from build123d import *

# Parameters (mm, degrees)
F0_W     = 31.75
F0_H     = 31.75
F0_W_2   = 9.525
F0_H_2   = 50.8
F0_R     = 3.175
F0_R_2   = 6.35
F1_DEPTH = 12.7
F2_R     = 3.175
F3_W     = 9.525
F3_H     = 38.1
F4_DEPTH = 1.5875
F5_W     = 9.525
F5_H     = 12.7
F6_DEPTH = 1.5875
F7_W     = 9.525
F7_H     = 50.8
F8_DEPTH = 1.5875
F9_R     = 6.35


with BuildPart() as f1:
    # F0 (on Right) → F1 (new body)
    with BuildSketch(Plane.YZ):
        with BuildLine():
            Line((0, 41.275), (0, 0))
            Line((0, 0), (130.175, 0))
            Line((130.175, 0), (130.175, 50.8))
            Line((130.175, 50.8), (73.025, 50.8))
            Line((73.025, 50.8), (73.025, 44.45))
            ThreePointArc((73.025, 44.45), (76.2, 41.275), (73.025, 38.1))
            Line((73.025, 38.1), (63.5, 38.1))
            ThreePointArc((63.5, 38.1), (60.325, 41.275), (63.5, 44.45))
            Line((63.5, 44.45), (63.5, 50.8))
            Line((63.5, 50.8), (50.8, 50.8))
            Line((50.8, 50.8), (50.8, 25.4))
            ThreePointArc((50.8, 25.4), (44.45, 19.05), (38.1, 25.4))
            Line((38.1, 25.4), (38.1, 50.8))
            Line((38.1, 50.8), (26.7157145118, 50.8))
            Line((26.7157145118, 50.8), (0, 41.275))
        make_face()
        with Locations((104.775, 25.4)):
            Rectangle(F0_W, F0_H, mode=Mode.SUBTRACT)
        with Locations((134.9375, 25.4)):
            Rectangle(F0_W_2, F0_H_2)
        with BuildLine():
            Line((139.7, 50.8), (139.7, 0))
            Line((139.7, 0), (304.8, 0))
            Line((304.8, 0), (304.8, 19.05))
            Line((304.8, 19.05), (266.7, 19.05))
            Line((266.7, 19.05), (266.7, 40.9178125))
            Line((266.7, 40.9178125), (290.922752809, 52.7264044944))
            ThreePointArc((290.922752809, 52.7264044944), (299.6985955056, 78.197752809), (274.227247191, 86.9735955056))
            Line((274.227247191, 86.9735955056), (200.025, 50.8))
            Line((200.025, 50.8), (139.7, 50.8))
        make_face()
        with Locations((230.1875, 12.7)):
            Circle(F0_R, mode=Mode.SUBTRACT)
        with Locations((165.1, 25.4)):
            Rectangle(F0_W, F0_H, mode=Mode.SUBTRACT)
        with BuildLine():
            Line((190.5, 38.1), (200.025, 38.1))
            ThreePointArc((200.025, 38.1), (203.2, 34.925), (200.025, 31.75))
            Line((200.025, 31.75), (200.025, 19.05))
            ThreePointArc((200.025, 19.05), (203.2, 15.875), (200.025, 12.7))
            Line((200.025, 12.7), (190.5, 12.7))
            ThreePointArc((190.5, 12.7), (187.325, 15.875), (190.5, 19.05))
            Line((190.5, 19.05), (190.5, 31.75))
            ThreePointArc((190.5, 31.75), (187.325, 34.925), (190.5, 38.1))
        make_face(mode=Mode.SUBTRACT)
        with Locations((282.575, 69.85)):
            Circle(F0_R_2, mode=Mode.SUBTRACT)
    extrude(amount=F1_DEPTH)

    # F2
    f2_edges = [f1.edges().sort_by_distance(p)[0] for p in [
        (6.35, 200.025, 50.8),
        (6.35, 266.7, 40.917812),
        (6.35, 266.7, 19.05),
        (6.35, 304.8, 19.05),
        (6.35, 304.8, 0),
    ]]
    fillet(f2_edges, radius=F2_R)

    # F3 (on face) → F4 (cut)
    with BuildSketch(Plane.YZ.offset(12.7)):
        with Locations((68.2625, 19.05)):
            Rectangle(F3_W, F3_H)
    extrude(amount=-F4_DEPTH, mode=Mode.SUBTRACT)

    # F5 (on face) → F6 (cut)
    with BuildSketch(Plane.YZ.offset(12.7)):
        with Locations((195.2625, 6.35)):
            Rectangle(F5_W, F5_H)
        with BuildLine():
            ThreePointArc((199.2923076923, 50.8), (199.6611512097, 50.8214972713), (200.025, 50.8856979781))
            Line((200.025, 50.8856979781), (200.025, 52.109055835))
            Line((200.025, 52.109055835), (190.5, 52.109055835))
            Line((190.5, 52.109055835), (190.5, 50.8))
            Line((190.5, 50.8), (199.2923076923, 50.8))
        make_face()
        with BuildLine():
            Line((190.5, 38.1), (200.025, 38.1))
            Line((200.025, 38.1), (200.025, 50.8856979781))
            ThreePointArc((200.025, 50.8856979781), (199.6611512097, 50.8214972713), (199.2923076923, 50.8))
            Line((199.2923076923, 50.8), (190.5, 50.8))
            Line((190.5, 50.8), (190.5, 38.1))
        make_face()
    extrude(amount=-F6_DEPTH, mode=Mode.SUBTRACT)

    # F7 (on face) → F8 (cut)
    with BuildSketch(Plane.YZ.offset(12.7)):
        with Locations((134.9375, 25.4)):
            Rectangle(F7_W, F7_H)
    extrude(amount=-F8_DEPTH, mode=Mode.SUBTRACT)

    # F9
    f9_edges = [f1.edges().sort_by_distance(p)[0] for p in [
        (6.35, 88.9, 41.275),
        (6.35, 120.65, 41.275),
        (6.35, 180.975, 41.275),
        (6.35, 149.225, 41.275),
        (6.35, 149.225, 9.525),
        (6.35, 88.9, 9.525),
        (6.35, 180.975, 9.525),
        (6.35, 120.65, 9.525),
    ]]
    fillet(f9_edges, radius=F9_R)


solid = f1.part
Design review of the part built by this model. Coordinates are the model's own, in mm. A direction names the side the tool comes from. Coordinates: 2 decimals unless noted, no trailing zeros. Order: outer loops, then holes, each group sorted by start corner. A loop starts at its lowest first (then second) coordinate and runs counter-clockwise, first axis right, second up.
Item 1: Take a section at A-A, the plane y = 166.5. Write out the cut boundary in (x, z) (3 decimals).
Item 2: For line 1 (Z direction, x = 7.25, y = 175); line 2 (Z direction, x = 9, y = 62.5); line 3 (Y direction, x = 5.25, z = 72), list the stretches that pass through material, from the lowest coordinate up.
Item 3: For pin 1 Ø4 at (x, z) = (9, 63.5) entering from +Y; pin 2 Ø0.5 at (x, z) = (12, 28) entering from +Y; pin 3 Ø6.5 at (x, z) = (6, 23) entering from +Y, all flat-tipped, find the tip position at first contact; note any pin that passes through.
Item 4: The part is to be moulded in two halves that separate along Y. For faces 1 (the flat face through (12.7, 252, 35)), 2 (the flat face through (6, 63.5, 48)), say which applies: pulls with the +Y half, pulls with the -Y half, needs draft (parallel to the pull), parting line crosses it, or undercut.
Item 5: For faces 3 (the flat face through (6, 57, 50.8)), 4 (the flat face through (12.7, 165, 9)), 5 (the flat face through (6, 200.025, 25)), 6 (the flat face through (11.112, 195, 45)), 7 (the flat face through (6, 73.025, 48)), list the 3-axis set-ups (+Z, -Z, +X, -X, +Y, -Y) from which the entire face can be reached by the end or side of a thin tool; tool diameter is ignored.
Item 6: Take a section at D-D, the plane y = 56.5. Write out the cut boundary in (x, z).
Item 7: Take a section at B-B, the plane z = 66.5. Write out the cut boundary in (x, y).
Item 8: Take a section at C-C, the plane x = 8. Count the separate pieces of the cut face and the enclosed holes in it, then the cut area to 3 significant figures.
The answers:
1. outline: (0, 0) - (12.7, 0) - (12.7, 9.525) - (0, 9.525) - close; (0, 41.275) - (12.7, 41.275) - (12.7, 50.8) - (0, 50.8) - close
2. line 1: z = 0 to 9.54, 41.26 to 50.8
2. line 2: z = 0 to 38.26, 44.29 to 50.8
2. line 3: y = 243.51 to 276.6, 288.55 to 301.5
3. pin 1: stops at y = 301.12
3. pin 2: stops at y = 266.7
3. pin 3: stops at y = 267.89
4. face 1: needs draft
4. face 2: undercut
5. face 3: +Z, +X, -X, -Y
5. face 4: +Z, -Z, +X, +Y, -Y
5. face 5: +X, -X
5. face 6: +Z, -Z, +X
5. face 7: +Z, +X, -X
6. outline: (0, 0) - (12.7, 0) - (12.7, 50.8) - (0, 50.8) - close
7. outline: (0, 232.23) - (12.7, 232.23) - (12.7, 277.18) - (0, 277.18) - close; (0, 287.97) - (12.7, 287.97) - (12.7, 301.33) - (0, 301.33) - close
8. separate pieces: 1
8. enclosed holes: 5
8. area: 13,500 mm2
